```python
from build123d import *

# Parameters (mm, degrees)
BOSS_EXTRUDE1_DEPTH      = 6
SKETCH2_R                = 5
CUT_EXTRUDE1_DEPTH       = 107
BOSS_EXTRUDE2_DEPTH      = 3.5
BOSS_EXTRUDE2_DEPTH_BACK = 3.5
SKETCH3_R                = 15
SKETCH4_R                = 10.85
CUT_EXTRUDE2_DEPTH       = 19.5
CIRPATTERN1_COUNT        = 3
SKETCH6_R                = 5
BOSS_EXTRUDE3_DEPTH      = 34
CUT_EXTRUDE5_DEPTH       = 103.68939394
CUT_EXTRUDE5_DEPTH_BACK  = 103.68939394
SKETCH12_W               = 81.781179221
SKETCH12_H               = 82.49231991
CUT_EXTRUDE6_DEPTH       = 39.848263365
CUT_EXTRUDE6_DEPTH_BACK  = 39.848263365
SKETCH13_W               = 17.873677222
SKETCH13_H               = 13.388121455
SKETCH13_W_2             = 15.899401816
SKETCH13_H_2             = 11.800117324


with BuildPart() as part:
    # Sketch1 → Boss-Extrude1 (new body)
    with BuildSketch(Plane(origin=(0, 0, 0), x_dir=(1, 0, 0), z_dir=(0, 1, 0))):
        Polygon((-11.547005384, 40), (-40.414518843, -10), (-28.867513459, -30), (28.867513459, -30), (40.414518843, -10), (11.547005384, 40), align=None)
    extrude(amount=BOSS_EXTRUDE1_DEPTH)

    # Sketch2 → Cut-Extrude1 (cut)
    with BuildSketch(Plane(origin=(0, 6, 0), x_dir=(1, 0, 0), z_dir=(0, 1, 0))):
        with Locations(Location((0, 0, 0), (0, 0, 270))):
            Circle(SKETCH2_R)
    extrude(amount=-CUT_EXTRUDE1_DEPTH, mode=Mode.SUBTRACT)

    # Sketch3 → Boss-Extrude2 (add, two sides: drawn at the far end of the back side and taken through both)
    with BuildSketch(Plane(origin=(0, 0, 0), x_dir=(0, 0, -1), z_dir=(1, 0, 0)).offset(-BOSS_EXTRUDE2_DEPTH_BACK)):
        with Locations((54.454926612, 4.00688116)):
            Circle(SKETCH3_R)
    extrude(amount=BOSS_EXTRUDE2_DEPTH + BOSS_EXTRUDE2_DEPTH_BACK)

    # Sketch4 → Cut-Extrude2 (cut)
    with BuildSketch(Plane(origin=(3.5, 0, 0), x_dir=(0, 0, -1), z_dir=(1, 0, 0))):
        with Locations((54.454926612, 4.00688116)):
            Circle(SKETCH4_R)
    extrude(amount=-CUT_EXTRUDE2_DEPTH, mode=Mode.SUBTRACT)


with BuildPart() as cirpattern1_1:
    # CirPattern1: pattern copy
    add(part.part.rotate(Axis((0, 0, 0), (0, 1, 0)), 1 * 360 / CIRPATTERN1_COUNT))


with BuildPart() as cirpattern1_2:
    # CirPattern1: pattern copy
    add(part.part.rotate(Axis((0, 0, 0), (0, 1, 0)), 2 * 360 / CIRPATTERN1_COUNT))


with BuildPart() as part_1:
    add(part.part)

    add(cirpattern1_1.part)  # Boss-Extrude3 merges CirPattern1_1

    add(cirpattern1_2.part)  # Boss-Extrude3 merges CirPattern1_2
    # Sketch6 → Boss-Extrude3 (add)
    with BuildSketch(Plane(origin=(0, 6, 0), x_dir=(1, 0, 0), z_dir=(0, 1, 0))):
        with Locations(Location((0, 0, 0), (0, 0, 270))):
            Circle(SKETCH6_R)
    extrude(amount=-BOSS_EXTRUDE3_DEPTH)


with BuildPart() as body_2:
    # Sketch8 → Revolve1 (revolve)
    with BuildSketch(Plane(origin=(0, -28, 0), x_dir=(-1, 0, 0), z_dir=(0, -1, 0))):
        with BuildLine():
            Line((0, 10), (0, -10))
            ThreePointArc((0, -10), (10, 0), (0, 10))
        make_face()
    revolve(axis=Axis((0, -28, 0), (0, 0, -1)))


with BuildPart() as cut_extrude5_tool:
    # Sketch12 → Cut-Extrude5 (new, two sides: drawn at the far end of the back side and taken through both)
    with BuildSketch(Plane(origin=(3.5, 0, 0), x_dir=(0, 0, -1), z_dir=(1, 0, 0)).offset(-CUT_EXTRUDE5_DEPTH_BACK)):
        with Locations((-9.89058961, -10.029914937)):
            Rectangle(SKETCH12_W, SKETCH12_H)
    extrude(amount=CUT_EXTRUDE5_DEPTH + CUT_EXTRUDE5_DEPTH_BACK)


with BuildPart() as part_2:
    add(part_1.part)

    # Cut-Extrude5: cut by cut_extrude5_tool
    add(cut_extrude5_tool.part, mode=Mode.SUBTRACT)

    # Sketch13 → Cut-Extrude6 (cut, two sides: drawn at the far end of the back side and taken through both)
    with BuildSketch(Plane(origin=(0, 0, -40), x_dir=(-1, 0, 0), z_dir=(0, 0, -1)).offset(-CUT_EXTRUDE6_DEPTH_BACK)):
        with Locations((12.436838611, -0.694060728)):
            Rectangle(SKETCH13_W, SKETCH13_H)
        with Locations((-11.449700908, 0.099941338)):
            Rectangle(SKETCH13_W_2, SKETCH13_H_2)
    extrude(amount=CUT_EXTRUDE6_DEPTH + CUT_EXTRUDE6_DEPTH_BACK, mode=Mode.SUBTRACT)


with BuildPart() as body_2_1:
    add(body_2.part)

    # Cut-Extrude5: cut by cut_extrude5_tool
    add(cut_extrude5_tool.part, mode=Mode.SUBTRACT)


solid = part_2.part
```
Source: CAD feature listing. Evaluate the final solid. Frame: model axes, mm. A direction names the side the tool comes from. Give positions to 0.01 mm unless a question says otherwise; leave off trailing zeros. Loops run counter-clockwise (first coordinate to the right, second up) from the corner with the lowest first, then second, coordinate; pieces in that order, holes last. Notation, with made-up numbers: (14.5, 49.5) -> (63.5, 49.5) arc R21 ccw to (63.5, 67.5) -> close; hole circle Ø5 at (1, 61.25). An arc over 180 degrees is marked (long way). Use a Markdown table: item, result. Add a question column.
(1) First-contact query: pin 1 Ø3 at (y, z) = (-4.5, -39) entering from +X; pin 2 Ø1.5 at (x, z) = (-2.5, -58.5) entering from -Y; pin 3 Ø1 at (x, y) = (2, -3) entering from +Z; pin 4 Ø3 at (x, z) = (1.5, -55) entering from +Y. Flat tips, straight axial feed; report the tip coordinate or a pass-through.
(2) Section query C-C (x = 0.75). Output: boundary loops of the cut face in (y, z).
(3) Ray query, line 1 (Y direction, x = 0.25, z = -54); line 2 (Y direction, x = 2, z = -39); line 3 (Z direction, x = 2.5, y = 11). Return the intervals inside material, ascending.
(4) Section query A-A (y = 13). Output: boundary loops of the cut face in (x, z).
(5) Access query for faces 1 (the face through (0.049, 7.266, -64.804)), 2 (the face through (0, 6, -35)), 3 (the face through (0, 0, -36)). Directions: +Z, -Z, +X, -X, +Y, -Y. A direction counts if a zero-diameter tool reaches every point of the face in a straight line with its end or side. Return the directions, or none.
(6) Section query D-D (z = -36.5). Output: boundary loops of the cut face in (x, y), then the cut area to 3 significant figures.
(7) Section query B-B (z = -57.5). Output: boundary loops of the cut face in (x, y), then the cut area to 3 significant figures.
Checked values:
| question | item | result |
|---|---|---|
| 1 | pin 1 | through |
| 1 | pin 2 | y = -10.63 |
| 1 | pin 3 | z = -40.94 |
| 1 | pin 4 | y = 19.01 |
| 2 | outline | (0, -40) arc R15 ccw (long way) to (6, -39.59) -> (6, -31) -> (0, -31) -> close; hole circle Ø21.7 at (4.01, -54.45) |
| 3 | line 1 | -10.99 to -6.83, 14.85 to 19 |
| 3 | line 2 | 0 to 6 |
| 3 | line 3 | -67.73 to -62.75, -46.16 to -41.18 |
| 4 | outline | (-3.5, -66.46) -> (3.5, -66.46) -> (3.5, -60.53) -> (-3.5, -60.53) -> close; (-3.5, -48.38) -> (3.5, -48.38) -> (3.5, -42.45) -> (-3.5, -42.45) -> close |
| 5 | face 1 | +X, -X |
| 5 | face 2 | +Z, +X, -X, +Y |
| 5 | face 3 | +Z, +X, -X, -Y |
| 6 | outline | (-3.5, 0) -> (3.5, 0) -> (3.5, 6) -> (-3.5, 6) -> close |
| 6 | area | 42.0 mm^2 |
| 7 | outline | (-3.5, -10.68) -> (3.5, -10.68) -> (3.5, -6.41) -> (-3.5, -6.41) -> close; (-3.5, 14.42) -> (3.5, 14.42) -> (3.5, 18.69) -> (-3.5, 18.69) -> close |
| 7 | area | 59.8 mm^2 |
